Geometry: see drawing. Coordinates: mm, zero at the bounding-box minimum. A direction names the side the tool comes from. Coordinates: 2 decimals unless noted, no trailing zeros. Order: outer loops, then holes, each group sorted by start corner. A loop starts at its lowest first (then second) coordinate and runs counter-clockwise, first axis right, second up.
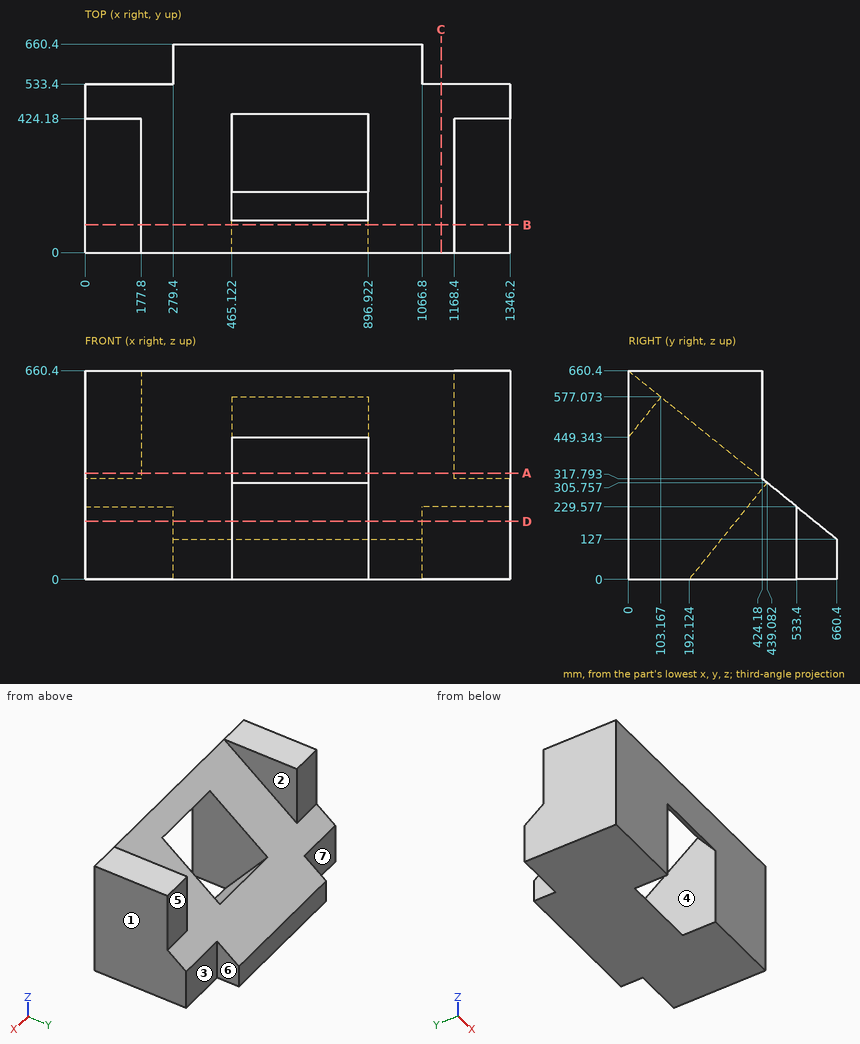
Q1. Material intervals for line 1 along X through (y, z) = (108.5, 474); line 2 along X through (y, z) = (192.5, 617.5); line 3 along Y through (x, z) = (156, 547.5), sorted ascending.
Solutions:
line 1: x = 0 to 465.12, 896.92 to 1346.2
line 2: x = 0 to 177.8, 1168.4 to 1346.2
line 3: y = 0 to 424.18
Q2. Section query A-A on z = 336. Output: boundary loops of the cut face in (x, y), plus the area to 3 significant figures.
Solutions:
outline: (0, 0) - (465.12, 0) - (465.12, 401.64) - (177.8, 401.64) - (177.8, 424.18) - (0, 424.18) - close; (896.92, 0) - (1346.2, 0) - (1346.2, 424.18) - (1168.4, 424.18) - (1168.4, 401.64) - (896.92, 401.64) - close
area: 375,000 mm2
Q3. Pull-direction query (X, two-part tool) for the marked faces 1, 2, 3 and 4; classes: pulls with the +X half, pulls with the -X half, needs draft (parallel to the pull), parting line crosses it, or undercut.
Solutions:
face 1: pulls with the +X half
face 2: undercut
face 3: needs draft
face 4: undercut
Q4. Pin query (flat end, axial travel): P1, Ø12, axis at x = 501.5, y = 569, coming from the +Z side; P2, Ø8, axis at x = 507.5, y = 398.5, coming from the +Z side (1 decimal). Return the tip coordinate at first contact, or that it passes through.
Solutions:
P1: stops at z = 205.67
P2: stops at z = 260.5
Q5. Section query C-C on x = 1127. Output: boundary loops of the cut face in (y, z), plus the area to 3 significant figures.
Solutions:
outline: (0, 0) - (533.4, 0) - (533.4, 229.58) - (0, 660.4) - close
area: 237,000 mm2
Q6. Section query D-D on z = 183. Output: boundary loops of the cut face in (x, y).
Solutions:
outline: (0, 0) - (465.12, 0) - (465.12, 339.93) - (896.92, 339.93) - (896.92, 0) - (1346.2, 0) - (1346.2, 533.4) - (1066.8, 533.4) - (1066.8, 591.07) - (279.4, 591.07) - (279.4, 533.4) - (0, 533.4) - close
Q7. Set-up query: the marked faces 5, 6 and 7. Return all of +Z, -Z, +X, -X, +Y, -Y with unobstructed straight access to the full face (end or side cutting, diameter ignored); none if empty.
Solutions:
face 5: +Z, +X, -X, +Y
face 6: +Z, -Z, +X, +Y
face 7: +Z, -Z, -X, +Y
Q8. Section query B-B on y = 88. Output: boundary loops of the cut face in (x, z) (1 decimal), plus the area to 3 significant figures.
Solutions:
outline: (0, 0) - (465.1, 0) - (465.1, 558.3) - (896.9, 558.3) - (896.9, 0) - (1346.2, 0) - (1346.2, 660.4) - (1168.4, 660.4) - (1168.4, 589.3) - (177.8, 589.3) - (177.8, 660.4) - (0, 660.4) - close
area: 578,000 mm2
